Read the model definition and answer for the solid it produces. Units are mm, in the model's axes. A direction names the side the tool comes from. Coordinates: 2 decimals unless noted, no trailing zeros. Order: outer loops, then holes, each group sorted by start corner. A loop starts at its lowest first (then second) coordinate and runs counter-clockwise, first axis right, second up. Notation, with made-up numbers: M 76,80.5 L 85,80.5 A14 cw 85,100.5 Z; hole C 52,55 d5. An arc over 180 degrees is marked long. Use a Markdown table: item, result. Add a question column.
1) For faces 1 (the face through (10, 55, 0)), 2 (the face through (2.958, 9.483, -0.26)), 3 (the face through (-14.7, 107.5, -0.1)), determine the directions among +Z, -Z, +X, -X, +Y, -Y from which every point of the face is accessible in a straight line to the end or side of a thin tool.
2) Find the intervals of material crossed by probe 1 along Y at (x, z) = (2.1, 0); probe 2 along X at (y, z) = (109, 0); probe 3 along Z at (x, y) = (1, 52), in increasing order. Write a range as [from, to].
3) Find section A-A on z = 0. Write down the section's boundary in (x, y), plus the area to 3 significant figures.
4) The mould has two halves that part along Z. Classify faces 4 (the face through (4, 55, 5)), 5 (the face through (-72.974, 110.035, -1.249)), 6 (the face through (6, 8, 0)): released by +Z, released by -Z, zero draft, split by the parting line, or undercut.
5) Each of these flat-tipped pins is pushed along its axis until it touches: pin 1 Ø11.5 at (x, y) = (-4.5, 35.5) entering from -Z; pin 2 Ø12 at (y, z) = (12, -7.5) entering from -X; pin 3 Ø1.2 at (y, z) = (7, 0) entering from -X; pin 4 Ø10 at (x, z) = (-5, 11) entering from +Y. Where does it stop, or does it pass through?
6) Find section D-D on x = 4. Write down the section's boundary in (y, z), plus the area to 3 significant figures.
7) Find section C-C on y = 7.5. Write down the section's boundary in (x, z), plus the area to 3 significant figures.
8) Find section B-B on x = -35. Write down the section's boundary in (y, z).
from build123d import *

# Parameters (mm, degrees)
ESQUISSE3_W             = 10
ESQUISSE3_H             = 70
BOSS_EXTRU_1_DEPTH      = 5
ESQUISSE8_R             = 30
ESQUISSE8_R_2           = 28
BOSS_EXTRU_4_DEPTH      = 2.5
ESQUISSE8_W             = 22
ESQUISSE8_H             = 10
BOSS_EXTRU_4_2_DEPTH    = 2.5
BOSS_EXTRU_5_REACH      = 107.494
ESQUISSE9_W             = 10
ESQUISSE9_H             = 10
BOSS_EXTRU_6_REACH      = 133.443
ESQUISSE10_W            = 10
ESQUISSE10_H            = 5
ESQUISSE11_R            = 2
ENL_V_MAT_EXTRU_1_DEPTH = 6


with BuildPart() as part:
    # Esquisse3 → Boss.-Extru.1 (new, symmetric)
    with BuildSketch(Plane.XY):
        with Locations((5, 35)):
            Rectangle(ESQUISSE3_W, ESQUISSE3_H)
    extrude(amount=BOSS_EXTRU_1_DEPTH, both=True)


with BuildPart() as body_2:
    # Esquisse8 → Boss.-Extru.4 (new, symmetric)
    with BuildSketch(Plane(origin=(0, 110, 0), x_dir=(1, 0, 0), z_dir=(0, 1, 0))):
        with Locations(Location((-43, 0, 0), (0, 0, 270))):
            Circle(ESQUISSE8_R)
        with Locations(Location((-43, 0, 0), (0, 0, 270))):
            Circle(ESQUISSE8_R_2, mode=Mode.SUBTRACT)
    extrude(amount=BOSS_EXTRU_4_DEPTH, both=True)

    # Esquisse10 → Boss.-Extru.6 (add, up to next)
    with BuildSketch(Plane.ZY.offset(12), mode=Mode.PRIVATE) as boss_extru_6_sk1:
        with Locations((0, 110)):
            Rectangle(ESQUISSE10_W, ESQUISSE10_H)
    boss_extru_6_tool1 = extrude(boss_extru_6_sk1.sketch, amount=BOSS_EXTRU_6_REACH, mode=Mode.PRIVATE) - body_2.part


with BuildPart() as body_3:
    # Esquisse8 → Boss.-Extru.4 2 (new, symmetric)
    with BuildSketch(Plane(origin=(0, 110, 0), x_dir=(1, 0, 0), z_dir=(0, 1, 0))):
        with Locations((-1, 0)):
            Rectangle(ESQUISSE8_W, ESQUISSE8_H)
    extrude(amount=BOSS_EXTRU_4_2_DEPTH, both=True)

    # Esquisse9 → Boss.-Extru.5 (add, up to next)
    with BuildSketch(Plane(origin=(0, 70, 0), x_dir=(1, 0, 0), z_dir=(0, 1, 0)), mode=Mode.PRIVATE) as boss_extru_5_sk1:
        with Locations((5, 0)):
            Rectangle(ESQUISSE9_W, ESQUISSE9_H)
    boss_extru_5_tool1 = extrude(boss_extru_5_sk1.sketch, amount=BOSS_EXTRU_5_REACH, mode=Mode.PRIVATE) - body_3.part

    add(part.part)  # Boss.-Extru.5 merges part
    add(boss_extru_5_tool1.solids().sort_by_distance((5, 70, 0))[0])


with BuildPart() as body_2_1:
    add(body_2.part)

    add(body_3.part)  # Boss.-Extru.6 merges body 3
    add(boss_extru_6_tool1.solids().sort_by_distance((-12, 110, 0))[0])

    # Esquisse11 → Enlèv. mat.-Extru.1 (cut)
    with BuildSketch(Plane.ZY):
        with Locations((0, 7.5)):
            Circle(ESQUISSE11_R)
    extrude(amount=-ENL_V_MAT_EXTRU_1_DEPTH, mode=Mode.SUBTRACT)


solid = body_2_1.part
Check result:
| question | item | result |
|---|---|---|
| 1 | face 1 | +Z, -Z, +X, +Y, -Y |
| 1 | face 2 | -X |
| 1 | face 3 | +Z, -Z, -X, -Y |
| 2 | probe 1 | y = [0, 5.5], [9.5, 112.5] |
| 2 | probe 2 | x = [-73, -71], [-15, 10] |
| 2 | probe 3 | z = [-5, 5] |
| 3 | outline | M -73,107.5 L -71,107.5 L -71,112.5 L -73,112.5 Z; M -15,107.5 L 0,107.5 L 0,9.5 L 6,9.5 L 6,5.5 L 0,5.5 L 0,0 L 10,0 L 10,112.5 L -15,112.5 Z |
| 3 | area | 1,190 mm2 |
| 4 | face 4 | released by +Z |
| 4 | face 5 | split by the parting line |
| 4 | face 6 | undercut |
| 5 | pin 1 | stops at z = -5 |
| 5 | pin 2 | stops at x = 0 |
| 5 | pin 3 | stops at x = 6 |
| 5 | pin 4 | passes through |
| 6 | outline | M 0,-5 L 112.5,-5 L 112.5,5 L 0,5 Z; hole C 7.5,0 d4 |
| 6 | area | 1,110 mm2 |
| 7 | outline | M 0,-5 L 10,-5 L 10,5 L 0,5 L 0,2 L 6,2 L 6,-2 L 0,-2 Z |
| 7 | area | 76.0 mm2 |
| 8 | outline | M 107.5,-28.91 L 112.5,-28.91 L 112.5,-26.83 L 107.5,-26.83 Z; M 107.5,26.83 L 112.5,26.83 L 112.5,28.91 L 107.5,28.91 Z |
